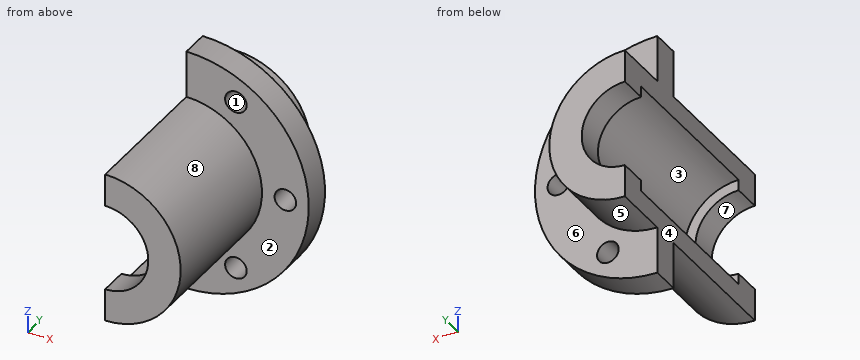
Autodesk Inventor part; units mm, degrees
ref_plane "YZ Plane" through (0, 0, 0) normal (1, 0, 0) x (0, 1, 0)
ref_plane "XZ Plane" through (0, 0, 0) normal (0, 1, 0) x (-1, 0, 0)
ref_plane "XY Plane" through (0, 0, 0) normal (0, 0, 1) x (1, 0, 0)
sketch "Sketch1" plane through (0, 0, 0) normal (0, 1, 0) x (-1, 0, 0)
  arc A0 (0, 7.5) -> (0, -7.5) centre (0, 0) ccw
  arc A1 (0, 10.5) -> (0, -10.5) centre (0, 0) ccw
  line L0 (0, 10.5) -> (0, 7.5)
  line L1 (0, -7.5) -> (0, -10.5)
  dimension "d0" = 7.5
  dimension "d1" = 3
extrude "Extrusion1" add sketch "Sketch1" along normal blind 24
sketch "Sketch2" plane through (0, 24, 0) normal (0, 1, 0) x (1, 0, 0)
  line L0 (0, 10.5) -> (0, 7.5)
  line L1 (0, -7.5) -> (0, -10.5)
  arc A0 (0, -10.5) -> (0, 10.5) centre (0, 0) ccw
  arc A1 (0, -6) -> (0, 6) centre (0, 0) ccw
  line L2 (0, 0) -> (0, 6) construction
  line L3 (0, 0) -> (6, 0) construction
  line L4 (0, 0) -> (0, -6) construction
  line L5 (0, 6) -> (0, 10.5)
  line L6 (0, -6) -> (0, -10.5)
  dimension "d6" = 6
  dimension "d7" = 90
  dimension "d8" = 180
extrude "Extrusion2" add sketch "Sketch2" along normal blind 4
sketch "Sketch3" plane through (0, 0, 0) normal (0, -1, 0) x (1, 0, 0)
  line L0 (0, -10.5) -> (0, -6)
  arc A0 (0, -6) -> (0, 6) centre (0, 0) ccw
  line L1 (0, 6) -> (0, 10.5)
  arc A1 (0, -10.5) -> (0, 10.5) centre (0, 0) ccw
extrude "Extrusion3" add sketch "Sketch3" along normal blind 4
ref_plane "Work Plane2" through (0, 16, 0) normal (0, 1, 0) x (1, 0, 0)
ref_plane "Work Plane1" through (0, 12, 0) normal (0, 1, 0) x (1, 0, 0)
sketch "Sketch5" plane through (0, 16, 0) normal (0, 1, 0) x (1, 0, 0)
  arc A0 (0, -10.5) -> (0, 10.5) centre (0, 0) ccw
  arc A1 (0, -17) -> (0, 17) centre (0, 0) ccw
  line L0 (0, 10.5) -> (0, 6)
  line L1 (0, 17) -> (0, 10.5)
  line L2 (0, -10.5) -> (0, -17)
  circle A2 centre (13.75, 0) radius 1.5
  line L3 (10.5, 0) -> (17, 0) construction
  circle A3 centre (6.875, 11.9078) radius 1.5
  circle A4 centre (6.875, -11.9078) radius 1.5
  dimension "d22" = 6.5
  dimension "d23" = 3
  dimension "d26" = 60
  dimension "d30" = 60
extrude "Extrusion4" add sketch "Sketch5" along normal blind 4
properties part number "Bearing_Holder" material "PC/ABS Plastic"
Check sheet for the modelled part. Datum: model origin and axes. Units: mm. Face numbers are marked on the shaded views. A direction names the side the tool comes from. Round coordinates to 2 decimals unless told otherwise and drop trailing zeros. Loops run counter-clockwise (first coordinate to the right, second up) from the corner with the lowest first, then second, coordinate; pieces in that order, holes last. Notation, with made-up numbers: (69.5, 40) - (111.5, 40) arc R29 cw to (111.5, 67) - close; hole circle Ø1 at (-20, -20). An arc over 180 degrees is marked (long way). Answer as CSV lines item,"result". Start each with the question number.
Item 1: Depth check by flat-ended pin: P1, Ø2.5, axis at x = 6.88, z = -11.91, coming from the +Y side; P2, Ø10, axis at y = 10, z = -9, coming from the +X side; P3, Ø2, axis at x = 4.5, y = 5.5, coming from the -Z side; P4, Ø6, axis at x = 15.5, z = 10, coming from the +Y side. Enter the tip coordinate at first touch or a pass-through.
Item 2: Section check B-B (x = 13.75). Record the boundary of the cut face in (y, z).
Item 3: Set-up check for the marked faces 1, 2, 3, 4 and 5: record each of +Z, -Z, +X, -X, +Y, -Y from which the full face is reachable in a straight line by a thin tool's end or side.
Item 4: Release check for a two-part mould opening along Z. For the marked faces 6, 7 and 8 record: +Z half, -Z half, draft (parallel to the pull), parting line (faces both ways), or undercut.
Item 5: Section check D-D (y = 7). Record the boundary of the cut face in (x, z).
Item 6: Scan lines: line 1 (Y direction, x = 3, z = -13); line 2 (Z direction, x = 6.25, y = 22); line 3 (Z direction, x = 13.75, y = 18.9). Record each from-to range of solid material in increasing order. Write a range as [from, to].
Item 7: Section check C-C (x = 10). Record the boundary of the cut face in (y, z).
Item 8: Section check A-A (z = 0). Record the boundary of the cut face in (x, y).
Report:
1,P1,"passes through"
1,P2,"stops at x = 9.71"
1,P3,"stops at z = -9.9"
1,P4,"stops at y = 20"
2,outline,"(16, -10) - (20, -10) - (20, -1.5) - (16, -1.5) - close; (16, 1.5) - (20, 1.5) - (20, 10) - (16, 10) - close"
3,face 1,"+Y, -Y"
3,face 2,"+X, -Y"
3,face 3,"-X"
3,face 4,"+Z, -Z, -X, +Y, -Y"
3,face 5,"+X, +Y"
4,face 6,"draft"
4,face 7,"undercut"
4,face 8,"parting line"
5,outline,"(0, -10.5) arc R10.5 ccw to (0, 10.5) - (0, 7.5) arc R7.5 cw to (0, -7.5) - close"
6,line 1,"y = [16, 20]"
6,line 2,"z = [-8.44, -4.15], [4.15, 8.44]"
6,line 3,"z = [-10, -1.5], [1.5, 10]"
7,outline,"(-4, -3.2) - (16, -3.2) - (16, -13.75) - (20, -13.75) - (20, -3.2) - (28, -3.2) - (28, 3.2) - (20, 3.2) - (20, 13.75) - (16, 13.75) - (16, 3.2) - (-4, 3.2) - close"
8,outline,"(6, -4) - (10.5, -4) - (10.5, 16) - (12.25, 16) - (12.25, 20) - (10.5, 20) - (10.5, 28) - (6, 28) - (6, 24) - (7.5, 24) - (7.5, 0) - (6, 0) - close; (15.25, 16) - (17, 16) - (17, 20) - (15.25, 20) - close"
